from build123d import *

# Parameters (mm, degrees)
SKETCH1_W            = 240
SKETCH1_H            = 300
BOSS_EXTRUDE1_DEPTH  = 370
SKETCH2_R            = 4.3
BOSS_EXTRUDE2_DEPTH  = 2.5
SKETCH3_W            = 204
SKETCH3_H            = 265
BOSS_EXTRUDE3_DEPTH  = 2.5
SKETCH8_R            = 4.286085294
BOSS_EXTRUDE6_DEPTH  = 2.5
SKETCH9_W            = 204
SKETCH9_H            = 265
BOSS_EXTRUDE7_DEPTH  = 2.5
SKETCH10_R           = 4.3
BOSS_EXTRUDE8_DEPTH  = 2.5
SKETCH12_W           = 204
SKETCH12_H           = 350
BOSS_EXTRUDE9_DEPTH  = 2.5
BOSS_EXTRUDE10_START = 2.5
SKETCH13_R           = 4.3
BOSS_EXTRUDE10_DEPTH = 2.5
SKETCH14_W           = 204
SKETCH14_H           = 350
BOSS_EXTRUDE11_DEPTH = 2.5
BOSS_EXTRUDE12_DEPTH = 1.5
BOSS_EXTRUDE13_DEPTH = 1.5


with BuildPart() as part:
    # Sketch1 → Boss-Extrude1 (new body)
    with BuildSketch(Plane(origin=(0, 0, 0), x_dir=(1, 0, 0), z_dir=(0, 1, 0))):
        Rectangle(SKETCH1_W, SKETCH1_H)
    extrude(amount=BOSS_EXTRUDE1_DEPTH)

    # Sketch2 → Boss-Extrude2 (add)
    with BuildSketch(Plane(origin=(0, 370, 0), x_dir=(1, 0, 0), z_dir=(0, 1, 0))):
        with Locations(Location((-86, 120, 0), (0, 0, 90))):
            Circle(SKETCH2_R)
        with Locations(Location((86, 120, 0), (0, 0, 90))):
            Circle(SKETCH2_R)
        with Locations(Location((86, -120, 0), (0, 0, 90))):
            Circle(SKETCH2_R)
        with Locations(Location((-86, -120, 0), (0, 0, 90))):
            Circle(SKETCH2_R)
    extrude(amount=BOSS_EXTRUDE2_DEPTH)

    # Sketch3 → Boss-Extrude3 (add)
    with BuildSketch(Plane(origin=(0, 372.5, 0), x_dir=(1, 0, 0), z_dir=(0, 1, 0))):
        Rectangle(SKETCH3_W, SKETCH3_H)
    extrude(amount=BOSS_EXTRUDE3_DEPTH)

    # Sketch8 → Boss-Extrude6 (add)
    with BuildSketch(Plane.XZ):
        with Locations(Location((-86, 120, 0), (0, 0, 270))):
            Circle(SKETCH8_R)
        with Locations(Location((86, 120, 0), (0, 0, 270))):
            Circle(SKETCH8_R)
        with Locations(Location((86, -120, 0), (0, 0, 270))):
            Circle(SKETCH8_R)
        with Locations(Location((-86, -120, 0), (0, 0, 270))):
            Circle(SKETCH8_R)
    extrude(amount=BOSS_EXTRUDE6_DEPTH)

    # Sketch9 → Boss-Extrude7 (add)
    with BuildSketch(Plane.XZ.offset(2.5)):
        Rectangle(SKETCH9_W, SKETCH9_H)
    extrude(amount=BOSS_EXTRUDE7_DEPTH)

    # Sketch10 → Boss-Extrude8 (add)
    with BuildSketch(Plane.XY.offset(150)):
        with Locations(Location((-86, 345, 0), (0, 0, 180))):
            Circle(SKETCH10_R)
        with Locations(Location((86, 345, 0), (0, 0, 180))):
            Circle(SKETCH10_R)
        with Locations(Location((86, 25, 0), (0, 0, 180))):
            Circle(SKETCH10_R)
        with Locations(Location((-86, 25, 0), (0, 0, 180))):
            Circle(SKETCH10_R)
    extrude(amount=BOSS_EXTRUDE8_DEPTH)

    # Sketch12 → Boss-Extrude9 (add)
    with BuildSketch(Plane.XY.offset(152.5)):
        with Locations((0, 185)):
            Rectangle(SKETCH12_W, SKETCH12_H)
    extrude(amount=BOSS_EXTRUDE9_DEPTH)

    # Sketch13 → Boss-Extrude10 (add)
    with BuildSketch(Plane(origin=(0, 0, -150), x_dir=(-1, 0, 0), z_dir=(0, 0, -1)).offset(BOSS_EXTRUDE10_START)):
        with Locations((-86, 345)):
            Circle(SKETCH13_R)
        with Locations((86, 345)):
            Circle(SKETCH13_R)
        with Locations((-86, 25)):
            Circle(SKETCH13_R)
        with Locations((86, 25)):
            Circle(SKETCH13_R)
    extrude(amount=-BOSS_EXTRUDE10_DEPTH)

    # Sketch14 → Boss-Extrude11 (add)
    with BuildSketch(Plane(origin=(0, 0, -152.5), x_dir=(-1, 0, 0), z_dir=(0, 0, -1))):
        with Locations((0, 185)):
            Rectangle(SKETCH14_W, SKETCH14_H)
    extrude(amount=BOSS_EXTRUDE11_DEPTH)

    # Sketch15 → Boss-Extrude12 (add)
    with BuildSketch(Plane.ZY.offset(120)):
        Polygon((-134.788231979, 161.45540947), (134.788231979, 161.45540947), (134.788231979, 35.45540947), (105.855505742, 11.598600117), (-105.855505742, 11.598600117), (-134.788231979, 35.45540947), align=None)
        Polygon((-134.788231979, 334.54459053), (-105.855505742, 358.401399883), (105.855505742, 358.401399883), (134.788231979, 334.54459053), (134.788231979, 208.54459053), (-134.788231979, 208.54459053), align=None)
    extrude(amount=BOSS_EXTRUDE12_DEPTH)

    # Sketch17 → Boss-Extrude13 (add)
    with BuildSketch(Plane(origin=(120, 0, 0), x_dir=(0, 0, -1), z_dir=(1, 0, 0))):
        Polygon((-134.788231979, 208.54459053), (134.788231979, 208.54459053), (134.788231979, 334.54459053), (105.855505742, 358.401399883), (-105.855505742, 358.401399883), (-134.788231979, 334.54459053), align=None)
        Polygon((-134.788231979, 161.45540947), (134.788231979, 161.45540947), (134.788231979, 35.45540947), (105.855505742, 11.598600117), (-105.855505742, 11.598600117), (-134.788231979, 35.45540947), align=None)
    extrude(amount=BOSS_EXTRUDE13_DEPTH)


solid = part.part
Geometry check sheet. Reference: the model listing, model coordinates, mm. A direction names the side the tool comes from. Coordinates: 2 decimals unless noted, no trailing zeros. Order: outer loops, then holes, each group sorted by start corner. A loop starts at its lowest first (then second) coordinate and runs counter-clockwise, first axis right, second up. Notation, with made-up numbers: (-25.5, 25) - (-16.5, 25) arc R24 cw to (-16.5, 38) - close; hole circle Ø6 at (-30, 21.25). An arc over 180 degrees is marked (long way). One line per item, written item: value.
(1) Release check for a two-part mould opening along X. For faces 5 (the face through (-1, 187, 155)), 6 (the face through (-87.984, 348.815, 151.232)) record: +X half, -X half, draft (parallel to the pull), parting line (faces both ways), or undercut.
Data:
face 5: draft
face 6: undercut
(2) Sectioned sample at A-A (y = 127.5). Enter the section's corners in (x, z).
Data:
outline: (-121.5, -134.79) - (-120, -134.79) - (-120, -150) - (120, -150) - (120, -134.79) - (121.5, -134.79) - (121.5, 134.79) - (120, 134.79) - (120, 150) - (-120, 150) - (-120, 134.79) - (-121.5, 134.79) - close; (-102, -155) - (102, -155) - (102, -152.5) - (-102, -152.5) - close; (-102, 152.5) - (102, 152.5) - (102, 155) - (-102, 155) - close
(3) Sectioned sample at C-C (x = -42.5). Enter the section's corners in (y, z).
Data:
outline: (-5, -132.5) - (-2.5, -132.5) - (-2.5, 132.5) - (-5, 132.5) - close; (0, -150) - (370, -150) - (370, 150) - (0, 150) - close; (10, -155) - (360, -155) - (360, -152.5) - (10, -152.5) - close; (10, 152.5) - (360, 152.5) - (360, 155) - (10, 155) - close; (372.5, -132.5) - (375, -132.5) - (375, 132.5) - (372.5, 132.5) - close
(4) Depth check by flat-ended pin: pin 1 Ø0.8 at (x, y) = (120.5, 250) entering from +Z; pin 2 Ø1.2 at (x, y) = (0, -3.5) entering from -Z; pin 3 Ø0.8 at (y, z) = (-4, -10.5) entering from +X. Enter the tip coordinate at first touch or a pass-through.
Data:
pin 1: stops at z = 134.79
pin 2: stops at z = -132.5
pin 3: stops at x = 102
(5) Thickness scan on probe 1 along Y at (x, z) = (95.5, 60); probe 2 along Z at (x, y) = (-3, 130); probe 3 along Y at (x, z) = (-109, -110). Record the ranges inside material, lowest first. Write a range as from..to.
Data:
probe 1: y = -5..-2.5, 0..370, 372.5..375
probe 2: z = -155..-152.5, -150..150, 152.5..155
probe 3: y = 0..370
(6) Sectioned sample at B-B (z = -84). Enter the section's corners in (x, y).
Data:
outline: (-121.5, 11.6) - (-120, 11.6) - (-120, 0) - (120, 0) - (120, 11.6) - (121.5, 11.6) - (121.5, 161.46) - (120, 161.46) - (120, 208.54) - (121.5, 208.54) - (121.5, 358.4) - (120, 358.4) - (120, 370) - (-120, 370) - (-120, 358.4) - (-121.5, 358.4) - (-121.5, 208.54) - (-120, 208.54) - (-120, 161.46) - (-121.5, 161.46) - close; (-102, -5) - (102, -5) - (102, -2.5) - (-102, -2.5) - close; (-102, 372.5) - (102, 372.5) - (102, 375) - (-102, 375) - close
(7) Access from +Z, -Z, +X, -X, +Y, -Y to the whole of each face (thin tool, end or side, straight path). Record for faces 1 (the face through (120.74, 23.36, 120.12)), 2 (the face through (81.9, 23.7, 151.2)), 3 (the face through (120.74, 346.64, 120.12)), 4 (the face through (-120.74, 23.36, -120.12)).
Data:
face 1: +Z, +X, -Y
face 2: none
face 3: +Z, +X, +Y
face 4: -Z, -X, -Y
